from build123d import *

# Parameters (mm, degrees)
SKETCH1_W           = 350
SKETCH1_H           = 50
BASE_FLANGE1_DEPTH  = 5
CUT_EXTRUDE1_REACH  = 178.847
SKETCH3_R           = 1.15
BREAK_CORNER2_START = -5
BREAK_CORNER2_DEPTH = 5


# Read off the part's stored shape, not the designer's step: Break-Corner2
# Sheet-metal steps are written as plain solids
with BuildPart() as part:
    # Sketch1 → Base-Flange1 (new body)
    with BuildSketch(Plane.XY):
        Rectangle(SKETCH1_W, SKETCH1_H)
        with BuildLine():
            Line((-167.75, -7.75), (-162.25, -7.75))
            ThreePointArc((-162.25, -7.75), (-160, -10), (-162.25, -12.25))
            Line((-162.25, -12.25), (-167.75, -12.25))
            ThreePointArc((-167.75, -12.25), (-170, -10), (-167.75, -7.75))
        make_face(mode=Mode.SUBTRACT)
        with BuildLine():
            Line((-167.75, 12.25), (-162.25, 12.25))
            ThreePointArc((-162.25, 12.25), (-160, 10), (-162.25, 7.75))
            Line((-162.25, 7.75), (-167.75, 7.75))
            ThreePointArc((-167.75, 7.75), (-170, 10), (-167.75, 12.25))
        make_face(mode=Mode.SUBTRACT)
        with BuildLine():
            Line((162.25, 12.25), (167.75, 12.25))
            ThreePointArc((167.75, 12.25), (170, 10), (167.75, 7.75))
            Line((167.75, 7.75), (162.25, 7.75))
            ThreePointArc((162.25, 7.75), (160, 10), (162.25, 12.25))
        make_face(mode=Mode.SUBTRACT)
        with BuildLine():
            Line((162.25, -7.75), (167.75, -7.75))
            ThreePointArc((167.75, -7.75), (170, -10), (167.75, -12.25))
            Line((167.75, -12.25), (162.25, -12.25))
            ThreePointArc((162.25, -12.25), (160, -10), (162.25, -7.75))
        make_face(mode=Mode.SUBTRACT)
    extrude(amount=-BASE_FLANGE1_DEPTH)

    # Sketch3 → Cut-Extrude1 (cut, up to next)
    with BuildSketch(Plane.XY, mode=Mode.PRIVATE) as cut_extrude1_sk1:
        with Locations((-80.5, 13.5)):
            Circle(SKETCH3_R)
    cut_extrude1_tool1 = extrude(cut_extrude1_sk1.sketch, amount=-CUT_EXTRUDE1_REACH, mode=Mode.PRIVATE) & part.part
    # Sketch3 → Cut-Extrude1 (cut, up to next)
    with BuildSketch(Plane.XY, mode=Mode.PRIVATE) as cut_extrude1_sk2:
        with Locations((-72.5, 13.5)):
            Circle(SKETCH3_R)
    cut_extrude1_tool2 = extrude(cut_extrude1_sk2.sketch, amount=-CUT_EXTRUDE1_REACH, mode=Mode.PRIVATE) & part.part
    # Sketch3 → Cut-Extrude1 (cut, up to next)
    with BuildSketch(Plane.XY, mode=Mode.PRIVATE) as cut_extrude1_sk3:
        with Locations((-64.5, 13.5)):
            Circle(SKETCH3_R)
    cut_extrude1_tool3 = extrude(cut_extrude1_sk3.sketch, amount=-CUT_EXTRUDE1_REACH, mode=Mode.PRIVATE) & part.part
    # Sketch3 → Cut-Extrude1 (cut, up to next)
    with BuildSketch(Plane.XY, mode=Mode.PRIVATE) as cut_extrude1_sk4:
        with Locations((-56.5, 13.5)):
            Circle(SKETCH3_R)
    cut_extrude1_tool4 = extrude(cut_extrude1_sk4.sketch, amount=-CUT_EXTRUDE1_REACH, mode=Mode.PRIVATE) & part.part
    # Sketch3 → Cut-Extrude1 (cut, up to next)
    with BuildSketch(Plane.XY, mode=Mode.PRIVATE) as cut_extrude1_sk5:
        with Locations((-86, -8)):
            Circle(SKETCH3_R)
    cut_extrude1_tool5 = extrude(cut_extrude1_sk5.sketch, amount=-CUT_EXTRUDE1_REACH, mode=Mode.PRIVATE) & part.part
    # Sketch3 → Cut-Extrude1 (cut, up to next)
    with BuildSketch(Plane.XY, mode=Mode.PRIVATE) as cut_extrude1_sk6:
        with Locations((-80.5, -13.5)):
            Circle(SKETCH3_R)
    cut_extrude1_tool6 = extrude(cut_extrude1_sk6.sketch, amount=-CUT_EXTRUDE1_REACH, mode=Mode.PRIVATE) & part.part
    # Sketch3 → Cut-Extrude1 (cut, up to next)
    with BuildSketch(Plane.XY, mode=Mode.PRIVATE) as cut_extrude1_sk7:
        with Locations((-72.5, -13.5)):
            Circle(SKETCH3_R)
    cut_extrude1_tool7 = extrude(cut_extrude1_sk7.sketch, amount=-CUT_EXTRUDE1_REACH, mode=Mode.PRIVATE) & part.part
    # Sketch3 → Cut-Extrude1 (cut, up to next)
    with BuildSketch(Plane.XY, mode=Mode.PRIVATE) as cut_extrude1_sk8:
        with Locations((-64.5, -13.5)):
            Circle(SKETCH3_R)
    cut_extrude1_tool8 = extrude(cut_extrude1_sk8.sketch, amount=-CUT_EXTRUDE1_REACH, mode=Mode.PRIVATE) & part.part
    # Sketch3 → Cut-Extrude1 (cut, up to next)
    with BuildSketch(Plane.XY, mode=Mode.PRIVATE) as cut_extrude1_sk9:
        with Locations((-56.5, -13.5)):
            Circle(SKETCH3_R)
    cut_extrude1_tool9 = extrude(cut_extrude1_sk9.sketch, amount=-CUT_EXTRUDE1_REACH, mode=Mode.PRIVATE) & part.part
    # Sketch3 → Cut-Extrude1 (cut, up to next)
    with BuildSketch(Plane.XY, mode=Mode.PRIVATE) as cut_extrude1_sk10:
        with Locations((-86, 8)):
            Circle(SKETCH3_R)
    cut_extrude1_tool10 = extrude(cut_extrude1_sk10.sketch, amount=-CUT_EXTRUDE1_REACH, mode=Mode.PRIVATE) & part.part
    # Sketch3 → Cut-Extrude1 (cut, up to next)
    with BuildSketch(Plane.XY, mode=Mode.PRIVATE) as cut_extrude1_sk11:
        with Locations((86, -8)):
            Circle(SKETCH3_R)
    cut_extrude1_tool11 = extrude(cut_extrude1_sk11.sketch, amount=-CUT_EXTRUDE1_REACH, mode=Mode.PRIVATE) & part.part
    # Sketch3 → Cut-Extrude1 (cut, up to next)
    with BuildSketch(Plane.XY, mode=Mode.PRIVATE) as cut_extrude1_sk12:
        with Locations((86, 8)):
            Circle(SKETCH3_R)
    cut_extrude1_tool12 = extrude(cut_extrude1_sk12.sketch, amount=-CUT_EXTRUDE1_REACH, mode=Mode.PRIVATE) & part.part
    # Sketch3 → Cut-Extrude1 (cut, up to next)
    with BuildSketch(Plane.XY, mode=Mode.PRIVATE) as cut_extrude1_sk13:
        with Locations((56.5, -13.5)):
            Circle(SKETCH3_R)
    cut_extrude1_tool13 = extrude(cut_extrude1_sk13.sketch, amount=-CUT_EXTRUDE1_REACH, mode=Mode.PRIVATE) & part.part
    # Sketch3 → Cut-Extrude1 (cut, up to next)
    with BuildSketch(Plane.XY, mode=Mode.PRIVATE) as cut_extrude1_sk14:
        with Locations((64.5, -13.5)):
            Circle(SKETCH3_R)
    cut_extrude1_tool14 = extrude(cut_extrude1_sk14.sketch, amount=-CUT_EXTRUDE1_REACH, mode=Mode.PRIVATE) & part.part
    # Sketch3 → Cut-Extrude1 (cut, up to next)
    with BuildSketch(Plane.XY, mode=Mode.PRIVATE) as cut_extrude1_sk15:
        with Locations((72.5, -13.5)):
            Circle(SKETCH3_R)
    cut_extrude1_tool15 = extrude(cut_extrude1_sk15.sketch, amount=-CUT_EXTRUDE1_REACH, mode=Mode.PRIVATE) & part.part
    # Sketch3 → Cut-Extrude1 (cut, up to next)
    with BuildSketch(Plane.XY, mode=Mode.PRIVATE) as cut_extrude1_sk16:
        with Locations((80.5, -13.5)):
            Circle(SKETCH3_R)
    cut_extrude1_tool16 = extrude(cut_extrude1_sk16.sketch, amount=-CUT_EXTRUDE1_REACH, mode=Mode.PRIVATE) & part.part
    # Sketch3 → Cut-Extrude1 (cut, up to next)
    with BuildSketch(Plane.XY, mode=Mode.PRIVATE) as cut_extrude1_sk17:
        with Locations((56.5, 13.5)):
            Circle(SKETCH3_R)
    cut_extrude1_tool17 = extrude(cut_extrude1_sk17.sketch, amount=-CUT_EXTRUDE1_REACH, mode=Mode.PRIVATE) & part.part
    # Sketch3 → Cut-Extrude1 (cut, up to next)
    with BuildSketch(Plane.XY, mode=Mode.PRIVATE) as cut_extrude1_sk18:
        with Locations((64.5, 13.5)):
            Circle(SKETCH3_R)
    cut_extrude1_tool18 = extrude(cut_extrude1_sk18.sketch, amount=-CUT_EXTRUDE1_REACH, mode=Mode.PRIVATE) & part.part
    # Sketch3 → Cut-Extrude1 (cut, up to next)
    with BuildSketch(Plane.XY, mode=Mode.PRIVATE) as cut_extrude1_sk19:
        with Locations((72.5, 13.5)):
            Circle(SKETCH3_R)
    cut_extrude1_tool19 = extrude(cut_extrude1_sk19.sketch, amount=-CUT_EXTRUDE1_REACH, mode=Mode.PRIVATE) & part.part
    # Sketch3 → Cut-Extrude1 (cut, up to next)
    with BuildSketch(Plane.XY, mode=Mode.PRIVATE) as cut_extrude1_sk20:
        with Locations((80.5, 13.5)):
            Circle(SKETCH3_R)
    cut_extrude1_tool20 = extrude(cut_extrude1_sk20.sketch, amount=-CUT_EXTRUDE1_REACH, mode=Mode.PRIVATE) & part.part
    # Sketch3 → Cut-Extrude1 (cut, up to next)
    with BuildSketch(Plane.XY, mode=Mode.PRIVATE) as cut_extrude1_sk21:
        with BuildLine():
            Line((-83, 10.5), (-54.69041576, 10.5))
            ThreePointArc((-54.69041576, 10.5), (-38.5, 0), (-54.69041576, -10.5))
            Line((-54.69041576, -10.5), (-83, -10.5))
            Line((-83, -10.5), (-83, 10.5))
        make_face()
    cut_extrude1_tool21 = extrude(cut_extrude1_sk21.sketch, amount=-CUT_EXTRUDE1_REACH, mode=Mode.PRIVATE) & part.part
    # Sketch3 → Cut-Extrude1 (cut, up to next)
    with BuildSketch(Plane.XY, mode=Mode.PRIVATE) as cut_extrude1_sk22:
        with BuildLine():
            Line((83, -10.5), (54.69041576, -10.5))
            ThreePointArc((54.69041576, -10.5), (38.5, 0), (54.69041576, 10.5))
            Line((54.69041576, 10.5), (83, 10.5))
            Line((83, 10.5), (83, -10.5))
        make_face()
    cut_extrude1_tool22 = extrude(cut_extrude1_sk22.sketch, amount=-CUT_EXTRUDE1_REACH, mode=Mode.PRIVATE) & part.part
    add(cut_extrude1_tool1.solids().sort_by_distance((-80.5, 13.5, 0))[0], mode=Mode.SUBTRACT)
    add(cut_extrude1_tool2.solids().sort_by_distance((-72.5, 13.5, 0))[0], mode=Mode.SUBTRACT)
    add(cut_extrude1_tool3.solids().sort_by_distance((-64.5, 13.5, 0))[0], mode=Mode.SUBTRACT)
    add(cut_extrude1_tool4.solids().sort_by_distance((-56.5, 13.5, 0))[0], mode=Mode.SUBTRACT)
    add(cut_extrude1_tool5.solids().sort_by_distance((-86, -8, 0))[0], mode=Mode.SUBTRACT)
    add(cut_extrude1_tool6.solids().sort_by_distance((-80.5, -13.5, 0))[0], mode=Mode.SUBTRACT)
    add(cut_extrude1_tool7.solids().sort_by_distance((-72.5, -13.5, 0))[0], mode=Mode.SUBTRACT)
    add(cut_extrude1_tool8.solids().sort_by_distance((-64.5, -13.5, 0))[0], mode=Mode.SUBTRACT)
    add(cut_extrude1_tool9.solids().sort_by_distance((-56.5, -13.5, 0))[0], mode=Mode.SUBTRACT)
    add(cut_extrude1_tool10.solids().sort_by_distance((-86, 8, 0))[0], mode=Mode.SUBTRACT)
    add(cut_extrude1_tool11.solids().sort_by_distance((86, -8, 0))[0], mode=Mode.SUBTRACT)
    add(cut_extrude1_tool12.solids().sort_by_distance((86, 8, 0))[0], mode=Mode.SUBTRACT)
    add(cut_extrude1_tool13.solids().sort_by_distance((56.5, -13.5, 0))[0], mode=Mode.SUBTRACT)
    add(cut_extrude1_tool14.solids().sort_by_distance((64.5, -13.5, 0))[0], mode=Mode.SUBTRACT)
    add(cut_extrude1_tool15.solids().sort_by_distance((72.5, -13.5, 0))[0], mode=Mode.SUBTRACT)
    add(cut_extrude1_tool16.solids().sort_by_distance((80.5, -13.5, 0))[0], mode=Mode.SUBTRACT)
    add(cut_extrude1_tool17.solids().sort_by_distance((56.5, 13.5, 0))[0], mode=Mode.SUBTRACT)
    add(cut_extrude1_tool18.solids().sort_by_distance((64.5, 13.5, 0))[0], mode=Mode.SUBTRACT)
    add(cut_extrude1_tool19.solids().sort_by_distance((72.5, 13.5, 0))[0], mode=Mode.SUBTRACT)
    add(cut_extrude1_tool20.solids().sort_by_distance((80.5, 13.5, 0))[0], mode=Mode.SUBTRACT)
    add(cut_extrude1_tool21.solids().sort_by_distance((-61.500767, 0, 0))[0], mode=Mode.SUBTRACT)
    add(cut_extrude1_tool22.solids().sort_by_distance((61.500767, 0, 0))[0], mode=Mode.SUBTRACT)

    # Break-Corner2 outline → Break-Corner2 (cut)
    with BuildSketch(Plane.XY.offset(BREAK_CORNER2_START)):
        with BuildLine():
            ThreePointArc((175, -22), (174.121320344, -24.121320344), (172, -25))
            Line((172, -25), (175, -25))
            Line((175, -25), (175, -22))
        make_face()
        with BuildLine():
            Line((-175, -25), (-172, -25))
            ThreePointArc((-172, -25), (-174.121320344, -24.121320344), (-175, -22))
            Line((-175, -22), (-175, -25))
        make_face()
        with BuildLine():
            ThreePointArc((172, 25), (174.121320344, 24.121320344), (175, 22))
            Line((175, 22), (175, 25))
            Line((175, 25), (172, 25))
        make_face()
        with BuildLine():
            Line((-175, 25), (-175, 22))
            ThreePointArc((-175, 22), (-174.121320344, 24.121320344), (-172, 25))
            Line((-172, 25), (-175, 25))
        make_face()
    extrude(amount=BREAK_CORNER2_DEPTH, mode=Mode.SUBTRACT)


solid = part.part
The listing builds one solid part. Answer for the finished solid, in the listing's coordinates (mm). Give positions to 0.01 mm unless a question says otherwise; leave off trailing zeros. Write each loop counter-clockwise with the first axis right and the second up, starting at its lowest first coordinate (ties: lowest second). Pieces come first, ordered by that corner, then holes.
1) For a pull along X with two mould halves and no side action, classify faces 1 (the face through (-2, 0, -5)), 2 (the face through (38.504, -0.32, -2.465)) as pulls with the +X half, pulls with the -X half, needs draft (parallel to the pull), parting line crosses it, or undercut.
2) Given P1, Ø1.4, axis at x = 86, y = 8, coming from the -Z side, flat-ended and moving along its own axis, determine where the tip first touches the part or whether it passes through.
3) Section A-A (x = -50) is taken. Write down the section's boundary in (y, z).
4) Find the intervals of material crossed by L1, parallel to X at y = 0, z = -1.6; L2, parallel to Y at x = -86, z = -3.75; L3, parallel to Y at x = 64.5, z = -1.95, in increasing order.
5) Section C-C (z = -4.25) is taken. Count the separate pieces of the cut face and the enclosed holes in it, and give its area (3 significant figures).
6) Section B-B (y = 0) is taken. Write down the section's boundary in (x, z).
Response:
1. face 1: needs draft
1. face 2: undercut
2. P1: passes through
3. outline: (-25, -5) - (-11.5, -5) - (-11.5, 0) - (-25, 0) - close; (11.5, -5) - (25, -5) - (25, 0) - (11.5, 0) - close
4. L1: x = -175 to -83, -38.5 to 38.5, 83 to 175
4. L2: y = -25 to -9.15, -6.85 to 6.85, 9.15 to 25
4. L3: y = -25 to -14.65, -12.35 to -10.5, 10.5 to 12.35, 14.65 to 25
5. separate pieces: 1
5. enclosed holes: 26
5. area: 15,400 mm2
6. outline: (-175, -5) - (-83, -5) - (-83, 0) - (-175, 0) - close; (-38.5, -5) - (38.5, -5) - (38.5, 0) - (-38.5, 0) - close; (83, -5) - (175, -5) - (175, 0) - (83, 0) - close
